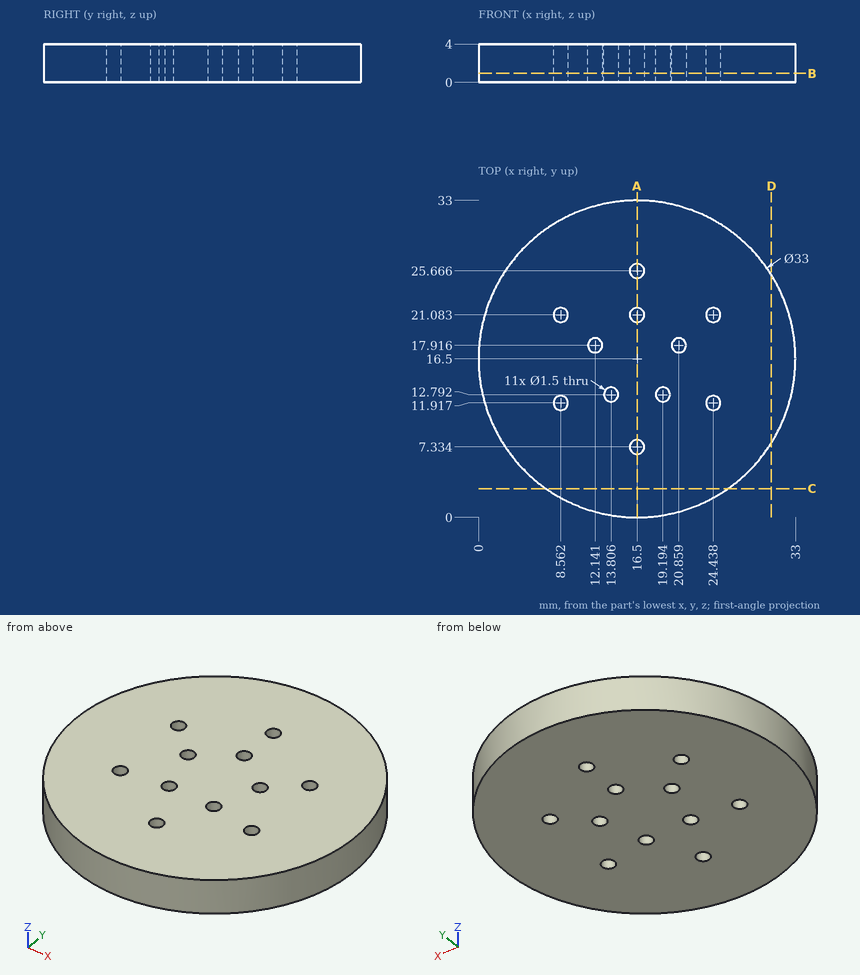
Source: three-view drawing plus pictorial views. Frame: mm from the lowest corner of the part. Round coordinates to 2 decimals unless told otherwise and drop trailing zeros. Loops run counter-clockwise (first coordinate to the right, second up) from the corner with the lowest first, then second, coordinate; pieces in that order, holes last. Notation, with made-up numbers: (-31.75, -10.5) - (-7.75, -10.5) arc R26 cw to (-7.75, 25.5) - close; hole circle Ø10 at (74, -36). An arc over 180 degrees is marked (long way). Write each question's results on one line, items separated by ' | '. Start each with the question number.
1) Cut plane B-B on z = 0.95. Count the separate pieces of the cut face and the enclosed holes in it, then the cut area to 3 significant figures.
2) Cut plane A-A on x = 16.5. Return loops of the section in (y, z).
3) Cut plane C-C on y = 3. Return loops of the section in (x, z).
4) Line query: probe 1 along Y at (x, z) = (16.5, 3.1); probe 2 along X at (y, z) = (21, 1.75) (1 decimal); probe 3 along Y at (x, z) = (17, 1.65) (1 decimal). Output: solid intervals per line, ascending. Write a range as [from, to].
5) Cut plane D-D on x = 30.5. Return loops of the section in (y, z).
6) First-contact query: P1, Ø1.2, axis at x = 16.5, y = 7.33, coming from the +Z side; P2, Ø1.7, axis at x = 24.44, y = 11.92, coming from the -Z side. Flat tips, straight axial feed; report the tip coordinate or a pass-through.
Verdict:
1) separate pieces: 1 | enclosed holes: 11 | area: 836 mm2
2) outline: (0, 0) - (6.58, 0) - (6.58, 4) - (0, 4) - close; (8.08, 0) - (20.33, 0) - (20.33, 4) - (8.08, 4) - close; (21.83, 0) - (24.92, 0) - (24.92, 4) - (21.83, 4) - close; (26.42, 0) - (33, 0) - (33, 4) - (26.42, 4) - close
3) outline: (7.01, 0) - (25.99, 0) - (25.99, 4) - (7.01, 4) - close
4) probe 1: y = [0, 6.58], [8.08, 20.33], [21.83, 24.92], [26.42, 33] | probe 2: x = [0.6, 7.8], [9.3, 15.8], [17.2, 23.7], [25.2, 32.4] | probe 3: y = [0, 6.8], [7.9, 20.5], [21.6, 25.1], [26.2, 33]
5) outline: (7.77, 0) - (25.23, 0) - (25.23, 4) - (7.77, 4) - close
6) P1: passes through | P2: stops at z = 0
